Could you check a few things on this drawing? It's one solid part, dimensions in mm from its lowest x, y, z. A direction names the side the tool comes from. Coordinates: 2 decimals unless noted, no trailing zeros. Write each loop counter-clockwise with the first axis right and the second up, starting at its lowest first coordinate (ties: lowest second). Pieces come first, ordered by that corner, then holes. Notation, with made-up numbers: (-13.5, 20) - (30.5, 20) arc R23 ccw to (30.5, 30) - close; hole circle Ø1 at (42.5, -14). An arc over 180 degrees is marked (long way). Write each question's results on one line, items separated by ' | '. Start each with the question number.
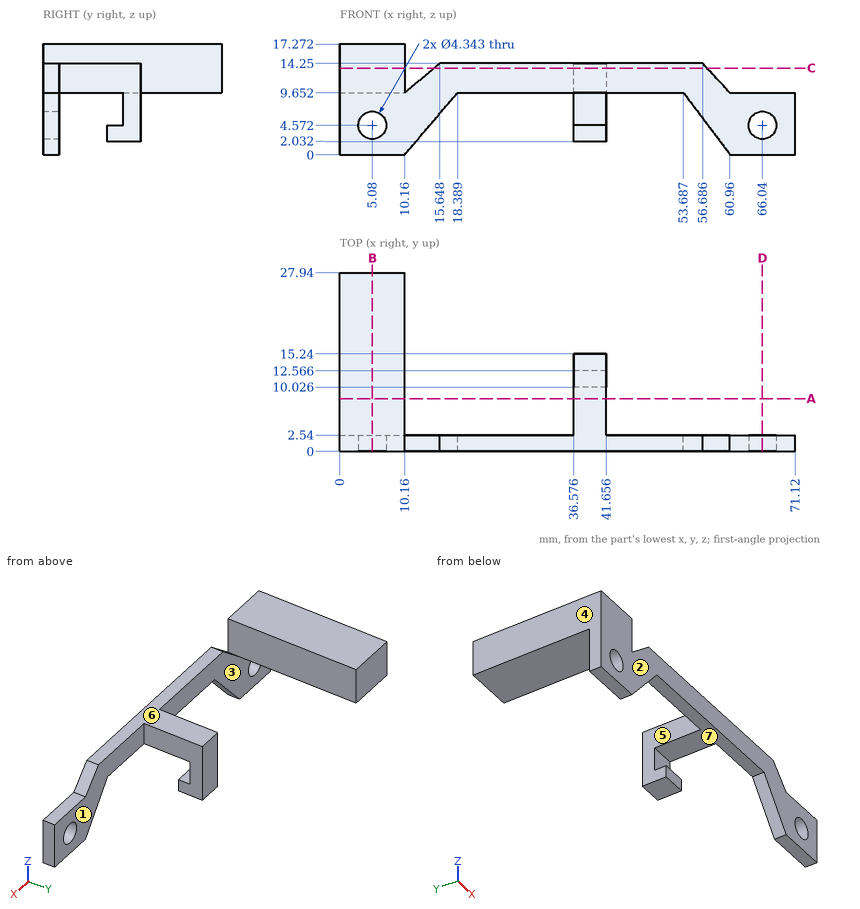
Q1. I'm going to push flat-ended pins straight in: pin 1 Ø1.5 at (x, z) = (38, 8) entering from -Y; pin 2 Ø4 at (y, z) = (19, 13.5) entering from +X; pin 3 Ø6.5 at (x, y) = (35, 3.5) entering from -Z; pin 4 Ø3 at (x, z) = (64, 8.5) entering from -Y. Where does each tip first touch, or does it pass through?
Q2. Thinking about a two-plate mould opening in X: for the marked faces 4, 5, 6 and 7, which applies, pulls with the +X half, pulls with the -X half, needs draft (parallel to the pull), parting line crosses it, or undercut?
Q3. If we section it at A-A (y = 8.25): Please give me the cut outline in (x, z), then the cut area to 3 significant figures.
Q4. If we section it at B-B (x = 5.08): Please give me the cut outline in (y, z).
Q5. I need wall thicknesses on line 1 along Z through (x, y) = (66.04, 0.5); line 2 along X through (y, z) = (10.5, 10); line 3 along X through (y, z) = (1.75, 6.5) (1 decimal). Which ranges of each line are inside material? Lowest first, please. Write a range as from..to.
Q6. For the marked faces 1, 2 and 3, which set-ups out of +Z, -Z, +X, -X, +Y, -Y let a thin tool reach every point of the face, with its end or its side?
Q7. If we section it at C-C (z = 13.5): Please give me the cut outline in (x, y).
Q8. If we section it at D-D (x = 66.04): Please give me the cut outline in (y, z), then the cut area to 3 significant figures.
Answer list:
1) pin 1: stops at y = 12.57 | pin 2: stops at x = 10.16 | pin 3: stops at z = 9.65 | pin 4: stops at y = 0
2) face 4: pulls with the -X half | face 5: undercut | face 6: needs draft | face 7: undercut
3) outline: (0, 9.65) - (10.16, 9.65) - (10.16, 17.27) - (0, 17.27) - close; (36.58, 9.65) - (41.66, 9.65) - (41.66, 14.25) - (36.58, 14.25) - close | area: 101 mm2
4) outline: (0, 0) - (2.54, 0) - (2.54, 2.4) - (0, 2.4) - close; (0, 6.74) - (2.54, 6.74) - (2.54, 9.65) - (27.94, 9.65) - (27.94, 17.27) - (0, 17.27) - close
5) line 1: z = 0..2.4, 6.74..9.65 | line 2: x = 0..10.16, 36.58..41.66 | line 3: x = 0..4.1, 6.1..15.7, 56.1..65, 67..71.1
6) face 1: +Z, -Z, +X, +Y | face 2: +Z, -Z, +X, -X, -Y | face 3: -Z, +Y
7) outline: (0, 0) - (10.16, 0) - (10.16, 27.94) - (0, 27.94) - close; (14.75, 0) - (57.38, 0) - (57.38, 2.54) - (41.66, 2.54) - (41.66, 15.24) - (36.58, 15.24) - (36.58, 2.54) - (14.75, 2.54) - close
8) outline: (0, 0) - (2.54, 0) - (2.54, 2.4) - (0, 2.4) - close; (0, 6.74) - (2.54, 6.74) - (2.54, 9.65) - (0, 9.65) - close | area: 13.5 mm2
